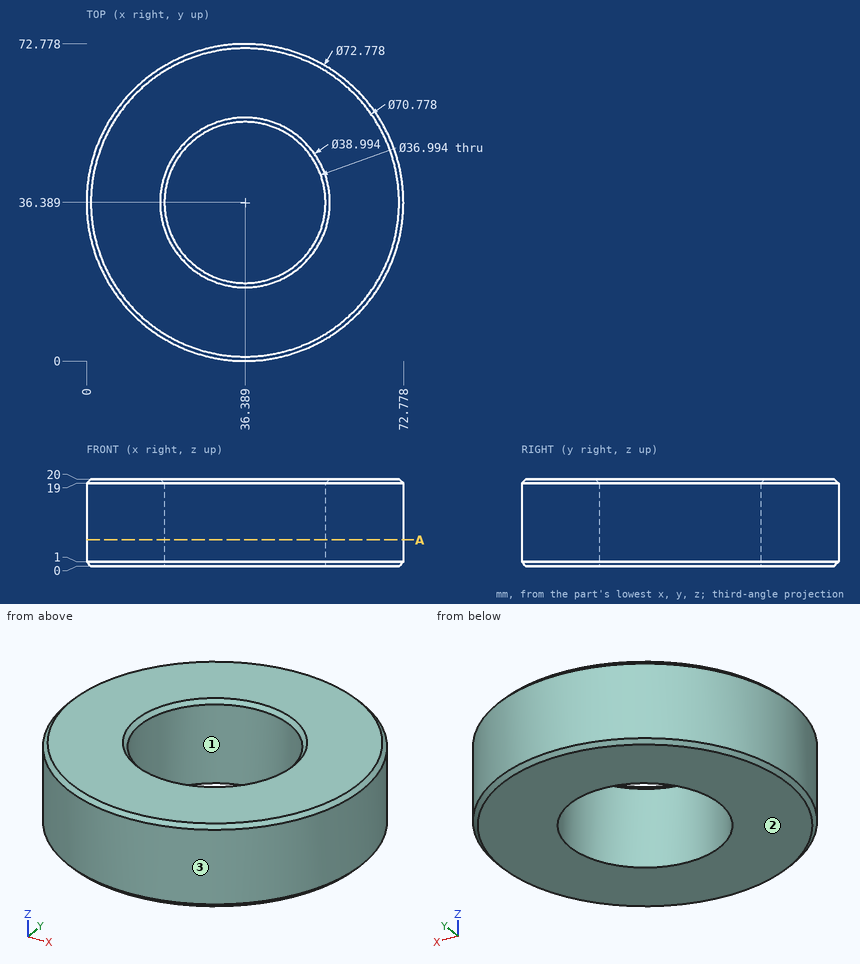
Verification items for this drawing (mm, ordinates from the low corner). Coordinates: 2 decimals unless noted, no trailing zeros. Loops run counter-clockwise (first coordinate to the right, second up) from the corner with the lowest first, then second, coordinate; pieces in that order, holes last. Notation, with made-up numbers: (67, 52) -> (92, 52) arc R23 ccw to (92, 84) -> close; hole circle Ø9 at (-39.5, -34.75). An arc over 180 degrees is marked (long way). Answer in a Markdown table with one row per item. Add a question column.
1. Draft check along X on the marked faces 1, 2 and 3. Enter one of: +X half, -X half, draft (parallel to the pull), parting line (faces both ways), or undercut.
2. Material ranges on probe 1 along Y at (x, z) = (36, 4.25) (1 decimal); probe 2 along Y at (x, z) = (22.5, 13.75) (1 decimal); probe 3 along X at (y, z) = (50, 15.5) (1 decimal), recorded low to high. Write a range as [from, to].
3. Section check A-A, the plane z = 6. Enter the section's corners in (x, y) (1 decimal).
4. Depth check by flat-ended pin: P1, Ø12, axis at x = 39, z = 4, coming from the -Y side; P2, Ø6, axis at y = 16, z = 9, coming from the +X side (1 decimal); P3, Ø2, axis at x = 58.5, z = 3, coming from the -Y side. Enter the tip coordinate at first touch or a pass-through.
Derived:
| question | item | result |
|---|---|---|
| 1 | face 1 | undercut |
| 1 | face 2 | draft |
| 1 | face 3 | parting line |
| 2 | probe 1 | y = [0, 17.9], [54.9, 72.8] |
| 2 | probe 2 | y = [2.8, 24.2], [48.6, 70] |
| 2 | probe 3 | x = [2.6, 23.9], [48.9, 70.1] |
| 3 | outline | circle Ø72.8 at (36.4, 36.4); hole circle Ø37 at (36.4, 36.4) |
| 4 | P1 | stops at y = 0 |
| 4 | P2 | stops at x = 68.4 |
| 4 | P3 | stops at y = 6.75 |
